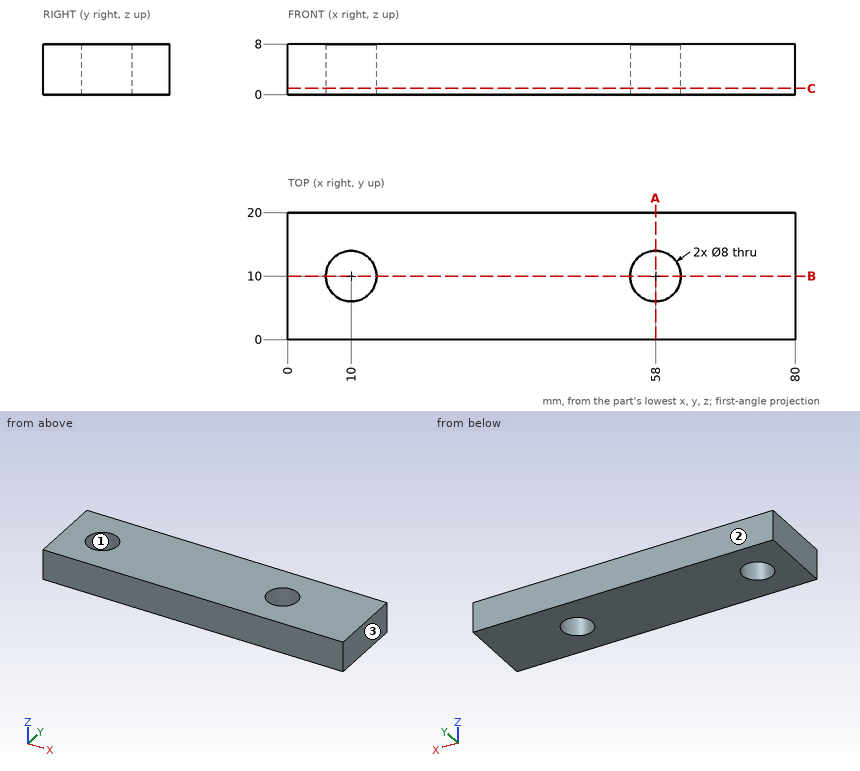
Part print with two shaded views. Sizes in mm from the minimum x, y, z corner. Round coordinates to 2 decimals unless told otherwise and drop trailing zeros. Order: outer loops, then holes, each group sorted by start corner. A loop starts at its lowest first (then second) coordinate and runs counter-clockwise, first axis right, second up.
(1) Drill centre lines: line 1 (X direction, y = 10, z = 6.25); line 2 (Y direction, x = 10, z = 5); line 3 (X direction, y = 10.75, z = 4). Where is each one in solid material? Low to high.
(2) Band-saw the part on C-C (z = 1). List the corners of the cut face in (x, y).
(3) Band-saw the part on A-A (x = 58). List the corners of the cut face in (y, z), then the cut area to 3 significant figures.
(4) Band-saw the part on B-B (y = 10). List the corners of the cut face in (x, z), then the cut area to 3 significant figures.
(5) Pull direction Y, two halves, no side cores. Call the marked faces 1, 2 and 3: released by +Y, released by -Y, zero draft, split by the parting line, or undercut.
Verdict:
1. line 1: x = 0 to 6, 14 to 54, 62 to 80
1. line 2: y = 0 to 6, 14 to 20
1. line 3: x = 0 to 6.07, 13.93 to 54.07, 61.93 to 80
2. outline: (0, 0) - (80, 0) - (80, 20) - (0, 20) - close; hole circle Ø8 at (10, 10); hole circle Ø8 at (58, 10)
3. outline: (0, 0) - (6, 0) - (6, 8) - (0, 8) - close; (14, 0) - (20, 0) - (20, 8) - (14, 8) - close
3. area: 96.0 mm2
4. outline: (0, 0) - (6, 0) - (6, 8) - (0, 8) - close; (14, 0) - (54, 0) - (54, 8) - (14, 8) - close; (62, 0) - (80, 0) - (80, 8) - (62, 8) - close
4. area: 512 mm2
5. face 1: undercut
5. face 2: released by +Y
5. face 3: zero draft
